For this review, take the finished solid that the model builds, in its own axes (mm). A direction names the side the tool comes from. Round coordinates to 2 decimals unless told otherwise and drop trailing zeros. Order: outer loops, then holes, each group sorted by start corner. A loop starts at its lowest first (then second) coordinate and runs counter-clockwise, first axis right, second up. Notation, with made-up numbers: (-12.75, -3.75) - (5.25, -3.75) arc R19 ccw to (5.25, 11.25) - close; hole circle Ø11 at (76.5, 85.25). An arc over 180 degrees is marked (long way). Write each question's results on one line, items separated by ' | '. Start each with the question number.
(1) Take a section at B-B, the plane x = -8. Give the boundary of the cut face in (y, z), plus the area to 3 significant figures.
(2) Insertion check: pin 1 Ø6 at (x, y) = (-82, -9) entering from +Z; pin 2 Ø1 at (x, z) = (-20, 10) entering from -Y; pin 3 Ø8 at (x, z) = (-47.5, 12) entering from +Y. Each pin has a flat end and moves straight along its axis. Give the tip position at first contact, or say it passes through.
(3) Take a section at A-A, the plane y = -22. Give the boundary of the cut face in (x, z).
(4) For faces 5 (the flat face through (-6, -24, 22.352)), 6 (the flat face through (-56, -7.366, 9)), list the 3-axis set-ups (+Z, -Z, +X, -X, +Y, -Y) from which the entire face can be reached by the end or side of a thin tool; tool diameter is ignored.
(5) For L1, parallel to X at y = -1, z = 20.75; L2, parallel to X at y = -21, z = 10.5; L3, parallel to Z at x = -41, y = 7.5, list the stretches that pass through material, from the lowest coordinate up. Write a range as from..to.
(6) Draft analysis for pull direction Y (two halves, no side actions). For faces 1 (the cylindrical face through (-48.1, -11.7, 1.6)), 2 (the flat face through (-47.87, -11, 2)), 3 (the flat face through (-59, -15.24, 8)), 4 (the flat face through (-56, 17.641, 2)), state which applies: pulls with the +Y half, pulls with the -Y half, needs draft (parallel to the pull), parting line crosses it, or undercut.
(7) Take a section at C-C, the plane z = 20.75. Give the boundary of the cut face in (x, y), plus the area to 3 significant figures.
(8) Take a section at D-D, the plane x = -55. Give the boundary of the cut face in (y, z), plus the area to 3 significant figures.
```python
from build123d import *

# Parameters (mm, degrees)
F1_DEPTH = 22.352
F2_DEPTH = 3.302
F4_DEPTH = 15.24
F5_DEPTH = 7.366


with BuildPart() as f1:
    # F0 (on Top) → F1 (new body)
    with BuildSketch(Plane.XY):
        with BuildLine():
            ThreePointArc((10.3024817516, -11.647160165), (1.7494492179, 9.0016869774), (-18.8993979245, 17.5547195112))
            Line((-18.8993979245, 17.5547195112), (-18.8993979245, 5.1860932686))
            ThreePointArc((-18.8993979245, 5.1860932686), (-6.9964902722, 0.2557474873), (-2.0661444909, -11.647160165))
            ThreePointArc((-2.0661444909, -11.647160165), (-6.9964902722, -23.5500678174), (-18.8993979245, -28.4804135986))
            Line((-18.8993979245, -28.4804135986), (-18.8993979245, -40.8490398412))
            ThreePointArc((-18.8993979245, -40.8490398412), (1.7494492179, -32.2960073074), (10.3024817516, -11.647160165))
        make_face()
        with BuildLine():
            Line((-18.8993979245, 5.1860932686), (-18.8993979245, 17.5547195112))
            ThreePointArc((-18.8993979245, 17.5547195112), (-38.2082616966, 10.2598605465), (-47.8701137319, -7.9800901862))
            Line((-47.8701137319, -7.9800901862), (-47.8701137319, -15.3142301438))
            ThreePointArc((-47.8701137319, -15.3142301438), (-38.2082616966, -33.5541808765), (-18.8993979245, -40.8490398412))
            Line((-18.8993979245, -40.8490398412), (-18.8993979245, -28.4804135986))
            ThreePointArc((-18.8993979245, -28.4804135986), (-35.7326513582, -11.647160165), (-18.8993979245, 5.1860932686))
        make_face()
    extrude(amount=F1_DEPTH)

    # F0 (on Top) → F2 (join)
    with BuildSketch(Plane.XY):
        with BuildLine():
            Line((-18.8993979245, 17.6407303661), (-94.2506045103, 17.6407303661))
            Line((-94.2506045103, 17.6407303661), (-94.2506045103, -40.9350506961))
            Line((-94.2506045103, -40.9350506961), (-18.8993979245, -40.9350506961))
            Line((-18.8993979245, -40.9350506961), (-18.8993979245, -40.8490398412))
            ThreePointArc((-18.8993979245, -40.8490398412), (-38.2082616966, -33.5541808765), (-47.8701137319, -15.3142301438))
            Line((-47.8701137319, -15.3142301438), (-76.080955565, -15.3142301438))
            Line((-76.080955565, -15.3142301438), (-76.080955565, -6.896413397))
            Line((-76.080955565, -6.896413397), (-47.8701137319, -6.896413397))
            Line((-47.8701137319, -6.896413397), (-47.8701137319, -7.9800901862))
            ThreePointArc((-47.8701137319, -7.9800901862), (-38.2082616966, 10.2598605465), (-18.8993979245, 17.5547195112))
            Line((-18.8993979245, 17.5547195112), (-18.8993979245, 17.6407303661))
        make_face()
        with BuildLine():
            ThreePointArc((-47.8701137319, -15.3142301438), (-48.1012776007, -11.647160165), (-47.8701137319, -7.9800901862))
            Line((-47.8701137319, -7.9800901862), (-47.8701137319, -6.896413397))
            Line((-47.8701137319, -6.896413397), (-76.080955565, -6.896413397))
            Line((-76.080955565, -6.896413397), (-76.080955565, -15.3142301438))
            Line((-76.080955565, -15.3142301438), (-47.8701137319, -15.3142301438))
        make_face()
    extrude(amount=F2_DEPTH)

    # F3 (on Front) → F4 (join)
    with BuildSketch(Plane.XZ):
        Polygon((-47.818031162, 22.1061483026), (-76.1827602983, 3.543845145), (-47.818031162, 3.0327689167), align=None)
    extrude(amount=F4_DEPTH)

    # F5 (cut): a face of the model
    f5_faces = [f1.faces().sort_by_distance(p)[0] for p in [
        (-57.3064596084, 0, 9.6084828756),
    ]]
    extrude(f5_faces, amount=-F5_DEPTH, mode=Mode.SUBTRACT)


solid = f1.part
```
Results below:
1) outline: (-38.74, 0) - (-24.48, 0) - (-24.48, 22.35) - (-38.74, 22.35) - close; (1.18, 0) - (15.44, 0) - (15.44, 22.35) - (1.18, 22.35) - close | area: 638 mm^2
2) pin 1: stops at z = 3.3 | pin 2: stops at y = -40.84 | pin 3: stops at y = 4.09
3) outline: (-94.25, 0) - (-32.17, 0) - (-32.17, 22.35) - (-46.2, 22.35) - (-46.2, 3.3) - (-94.25, 3.3) - close; (-5.63, 0) - (8.41, 0) - (8.41, 22.35) - (-5.63, 22.35) - close
4) face 5: +Z, +X, -X, +Y, -Y | face 6: +Z, -X, +Y
5) L1: x = -46.09..-31.94, -5.86..8.29 | L2: x = -46.56..-32.9, -4.9..8.76 | L3: z = 0..3.3
6) face 1: undercut | face 2: undercut | face 3: pulls with the -Y half | face 4: pulls with the +Y half
7) outline: (-49.89, -15.24) - (-47.87, -15.24) - (-47.87, -15.31) arc R29.2 ccw (long way) to (-47.82, -7.59) - (-47.82, -7.37) - (-49.89, -7.37) - close; hole circle Ø33.67 at (-18.9, -11.65) | area: 1,800 mm^2
8) outline: (-40.94, 0) - (17.64, 0) - (17.64, 3.3) - (-7.37, 3.3) - (-7.37, 17.41) - (-15.24, 17.41) - (-15.24, 3.3) - (-40.94, 3.3) - close | area: 304 mm^2
